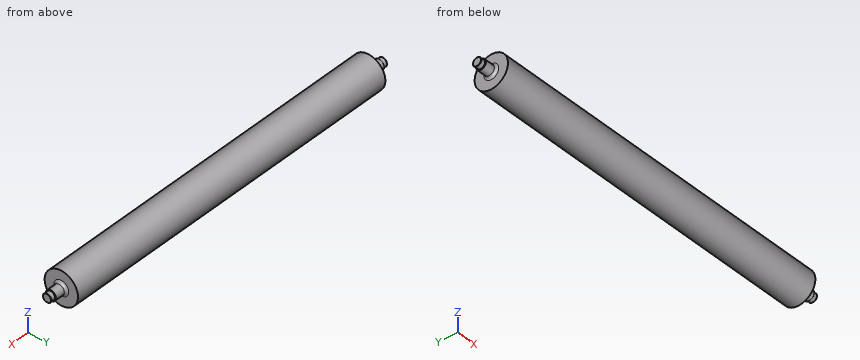
from build123d import *

# Parameters (mm, degrees)
F0_R     = 22.51329
F1_DEPTH = 1027.43
F2_R     = 27.0002
F3_DEPTH = 1003.554
F4_R     = 88.9
F5_DEPTH = 939.8
F6_R     = 12.7
F7_R     = 0.762
F8_R     = 0.762
F9_SIZE  = 1.524


with BuildPart() as f1:
    # F0 (on Right) → F1 (new body, symmetric)
    with BuildSketch(Plane.YZ):
        Circle(F0_R)
    extrude(amount=F1_DEPTH, both=True)

    # F2 (on Right) → F3 (join, symmetric)
    with BuildSketch(Plane.YZ):
        Circle(F2_R)
    extrude(amount=F3_DEPTH, both=True)

    # F4 (on Right) → F5 (join, symmetric)
    with BuildSketch(Plane.YZ):
        Circle(F4_R)
    extrude(amount=F5_DEPTH, both=True)

    # F6
    f6_edges = [f1.edges().sort_by_distance(p)[0] for p in [
        (939.8, -27.0002, 0),
        (-939.8, -27.0002, 0),
    ]]
    fillet(f6_edges, radius=F6_R)

    # F7
    f7_edges = [f1.edges().sort_by_distance(p)[0] for p in [
        (-1003.554, -22.51329, 0),
    ]]
    fillet(f7_edges, radius=F7_R)

    # F8
    f8_edges = [f1.edges().sort_by_distance(p)[0] for p in [
        (1003.554, -22.51329, 0),
    ]]
    fillet(f8_edges, radius=F8_R)

    # F9
    f9_edges = [f1.edges().sort_by_distance(p)[0] for p in [
        (1027.43, -22.51329, 0),
        (-1027.43, -22.51329, 0),
    ]]
    chamfer(f9_edges, length=F9_SIZE)


solid = f1.part
Input: part model. Units: mm. Frame: model coordinates. Give positions to 0.01 mm unless a question says otherwise; leave off trailing zeros. Order: outer loops, then holes, each group sorted by start corner. A loop starts at its lowest first (then second) coordinate and runs counter-clockwise, first axis right, second up. Notation, with made-up numbers: (27, 49.25) -> (77, 49.25) arc R10 ccw to (77, 54.25) -> close; hole circle Ø7 at (86.25, -34). An arc over 180 degrees is marked (long way). Use one line per item in the form item = value.
1) Line query: probe 1 along X at (y, z) = (73, -47.5); probe 2 along Y at (x, z) = (-435, -4); probe 3 along Z at (x, y) = (-525.5, -6). Output: solid intervals per line, ascending.
Response values:
probe_1 = -939.8 to 939.8
probe_2 = -88.81 to 88.81
probe_3 = -88.7 to 88.7
2) First-contact query: pin 1 Ø8 at (x, z) = (-747, -58.5) entering from -Y; pin 2 Ø6 at (y, z) = (38.5, 51.5) entering from -X; pin 3 Ø10 at (x, z) = (255.5, 19.5) entering from +Y. Flat tips, straight axial feed; report the tip coordinate or a pass-through.
Response values:
pin_1 = -70.24
pin_2 = -939.8
pin_3 = 87.71
3) Section C-C, the plane x = -680. Return loops of the section in (y, z), and give its area (3 significant figures).
Response values:
outline = circle Ø177.8 at (0, 0)
area = 24,800 mm^2
